Check sheet for the modelled part. Datum: model origin and axes. Units: mm. A direction names the side the tool comes from. Round coordinates to 2 decimals unless told otherwise and drop trailing zeros. Order: outer loops, then holes, each group sorted by start corner. A loop starts at its lowest first (then second) coordinate and runs counter-clockwise, first axis right, second up.
(1) Sectioned sample at B-B, the plane y = 0. Enter the section's corners in (x, z).
(2) Sectioned sample at D-D, the plane y = 6.25. Enter the section's corners in (x, z), and give its area (3 significant figures).
(3) Sectioned sample at C-C, the plane z = 30. Enter the section's corners in (x, y).
(4) Sectioned sample at A-A, the plane z = 37.5. Enter the section's corners in (x, y), and give its area (3 significant figures).
(5) Mould release check, pull along X, two halves, no side actions. Record for faces 6 (the flat face through (2, -7, 13)), 7 (the flat face through (-10, 0, 20)), 8 (the flat face through (10, 0, 20)): released by +X, released by -X, zero draft, split by the parting line, or undercut.
(6) Tool access check on faces 1 (the flat face through (-7, -10, 20)), 2 (the flat face through (7, -10, 20)), 3 (the cylindrical face through (-0.59, 4.46, 3.94)), 4 (the flat face through (2, -7, 28)), 5 (the flat face through (5, 0, 0)). Record the directions out of +Z, -Z, +X, -X, +Y, -Y that give a thin tool (end or side, any length) a straight path to the whole face; none if there is none.
(7) Thickness scan on probe 1 along X at (y, z) = (-8.9, 15); probe 2 along Z at (x, y) = (-1.25, -9); probe 3 along Y at (x, z) = (0, 8.5). Record the ranges inside material, lowest first.
(8) Depth check by flat-ended pin: pin 1 (5 mm diameter, centred on x = 0, z = 30, fed in from +Y); pin 2 (6 mm diameter, centred on x = 0, y = 0, fed in from +Z); pin 3 (4 mm diameter, centred on x = 0, y = 0, fed in from -Z); pin 4 (3 mm diameter, centred on x = -7.5, z = 17.5, fed in from -Y). Enter the tip coordinate at first touch or a pass-through.
```python
from build123d import *

# Parameters (mm, degrees)
PAD_DEPTH       = 40
SKETCH001_R     = 2.5
POCKET_DEPTH    = 40
SKETCH002_R     = 4.5
POCKET001_DEPTH = 8
SKETCH003_R     = 2.25
POCKET002_DEPTH = 22
SKETCH004_R     = 3.75
POCKET003_DEPTH = 17


with BuildPart() as part:
    # Sketch → Pad (new body)
    with BuildSketch(Plane.XY):
        Polygon((-10, -10), (-10, 10), (10, 10), (10, -10), (4.5, -10), (3.5, -11), (-3.5, -11), (-4.5, -10), align=None)
    extrude(amount=PAD_DEPTH)

    # Sketch001 → Pocket (cut)
    with BuildSketch(Plane.XY):
        Circle(SKETCH001_R)
    extrude(amount=POCKET_DEPTH, mode=Mode.SUBTRACT)

    # Sketch002 → Pocket001 (cut)
    with BuildSketch(Plane.XY):
        Circle(SKETCH002_R)
    extrude(amount=POCKET001_DEPTH, mode=Mode.SUBTRACT)

    # Sketch003 (on DatumPlane) → Pocket002 (cut)
    with BuildSketch(Plane.XZ.offset(-10)):
        with Locations((0, 15)):
            Circle(SKETCH003_R)
        with Locations((0, 30)):
            Circle(SKETCH003_R)
    extrude(amount=POCKET002_DEPTH, mode=Mode.SUBTRACT)

    # Sketch004 (on DatumPlane) → Pocket003 (cut)
    with BuildSketch(Plane.XZ.offset(-10)):
        with Locations((0, 30)):
            Circle(SKETCH004_R)
        with Locations((0, 15)):
            Circle(SKETCH004_R)
    extrude(amount=POCKET003_DEPTH, mode=Mode.SUBTRACT)


solid = part.part
```
Derived:
1. outline: (-10, 0) - (-4.5, 0) - (-4.5, 8) - (-2.5, 8) - (-2.5, 12.2) arc R3.75 cw to (-2.5, 17.8) - (-2.5, 27.2) arc R3.75 cw to (-2.5, 32.8) - (-2.5, 40) - (-10, 40) - close; (2.5, 8) - (4.5, 8) - (4.5, 0) - (10, 0) - (10, 40) - (2.5, 40) - (2.5, 32.8) arc R3.75 cw to (2.5, 27.2) - (2.5, 17.8) arc R3.75 cw to (2.5, 12.2) - close
2. outline: (-10, 0) - (10, 0) - (10, 40) - (-10, 40) - close; hole circle Ø7.5 at (0, 15); hole circle Ø7.5 at (0, 30)
2. area: 712 mm2
3. outline: (-10, -10) - (-4.5, -10) - (-3.5, -11) - (-2.25, -11) - (-2.25, -7) - (-3.75, -7) - (-3.75, 10) - (-10, 10) - close; (2.25, -11) - (3.5, -11) - (4.5, -10) - (10, -10) - (10, 10) - (3.75, 10) - (3.75, -7) - (2.25, -7) - close
4. outline: (-10, -10) - (-4.5, -10) - (-3.5, -11) - (3.5, -11) - (4.5, -10) - (10, -10) - (10, 10) - (-10, 10) - close; hole circle Ø5 at (0, 0)
4. area: 388 mm2
5. face 6: undercut
5. face 7: released by -X
5. face 8: released by +X
6. face 1: +Z, -Z, -X, -Y
6. face 2: +Z, -Z, +X, -Y
6. face 3: -Z
6. face 4: +Y
6. face 5: -Z, +X, -X, +Y, -Y
7. probe 1: x = -10 to -2.25, 2.25 to 10
7. probe 2: z = 0 to 13.13, 16.87 to 28.13, 31.87 to 40
7. probe 3: y = -11 to -2.5, 2.5 to 10
8. pin 1: stops at y = -7
8. pin 2: stops at z = 40
8. pin 3: passes through
8. pin 4: stops at y = -10
